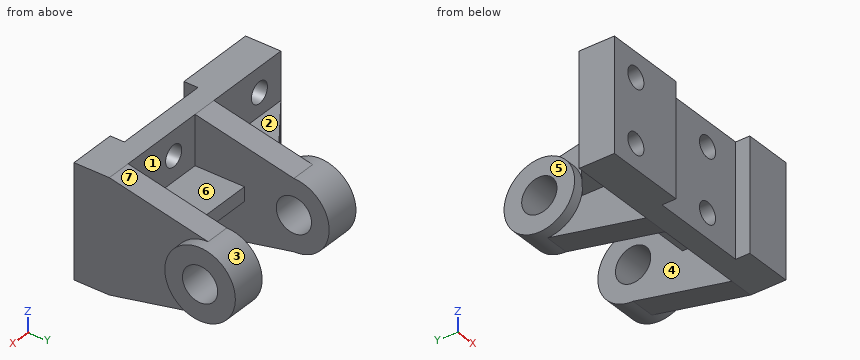
from build123d import *

# Parameters (mm, degrees)
SKETCH1_W           = 128
SKETCH1_H           = 64
BOSS_EXTRUDE1_DEPTH = 20
SKETCH2_W           = 55
SKETCH2_H           = 8
CUT_EXTRUDE1_DEPTH  = 93.69304181
SKETCH4_R           = 20
SKETCH4_R_2         = 10
BOSS_EXTRUDE3_DEPTH = 14
BOSS_EXTRUDE4_START = 6
SKETCH4_3_R         = 20
SKETCH4_3_R_2       = 10
BOSS_EXTRUDE4_DEPTH = 6
SKETCH18_W          = 50
SKETCH18_H          = 8
BOSS_EXTRUDE6_DEPTH = 28
RIB1_REACH          = 125.045
SKETCH19_WALL_W     = 309.701101848
SKETCH19_WALL_H     = 10
SKETCH20_R          = 6
CUT_EXTRUDE2_DEPTH  = 109.166538264
SKETCH21_R          = 6
CUT_EXTRUDE3_DEPTH  = 109.166538264
SKETCH22_R          = 6
CUT_EXTRUDE4_DEPTH  = 109.166538264


with BuildPart() as part:
    # Sketch1 → Boss-Extrude1 (new body)
    with BuildSketch(Plane(origin=(0, 0, 0), x_dir=(1, 0, 0), z_dir=(0, 1, 0))):
        Rectangle(SKETCH1_W, SKETCH1_H)
    extrude(amount=BOSS_EXTRUDE1_DEPTH)

    # Sketch2 → Cut-Extrude1 (cut, through all)
    with BuildSketch(Plane.XY.offset(32)):
        with Locations((9.5, 4)):
            Rectangle(SKETCH2_W, SKETCH2_H)
    extrude(amount=-CUT_EXTRUDE1_DEPTH, mode=Mode.SUBTRACT)

    # Sketch4 → Boss-Extrude3 (add)
    # profile 1 of 2: a face of its own
    with BuildSketch(Plane(origin=(64, 0, 0), x_dir=(0, 0, -1), z_dir=(1, 0, 0))):
        with BuildLine():
            ThreePointArc((20, 76), (0, 56), (-20, 76))
            Line((-20, 76), (-32, 20))
            Line((-32, 20), (32, 20))
            Line((32, 20), (20, 76))
        make_face()
    # profile 2 of 2: a face of its own
    with BuildSketch(Plane(origin=(64, 0, 0), x_dir=(0, 0, -1), z_dir=(1, 0, 0))):
        with Locations((0, 76)):
            Circle(SKETCH4_R)
        with Locations((0, 76)):
            Circle(SKETCH4_R_2, mode=Mode.SUBTRACT)
    boss_extrude3 = extrude(amount=-BOSS_EXTRUDE3_DEPTH)

    # Sketch4_3 → Boss-Extrude4 (add)
    with BuildSketch(Plane(origin=(64, 0, 0), x_dir=(0, 0, -1), z_dir=(1, 0, 0)).offset(BOSS_EXTRUDE4_START)):
        with Locations((0, 76)):
            Circle(SKETCH4_3_R)
        with Locations((0, 76)):
            Circle(SKETCH4_3_R_2, mode=Mode.SUBTRACT)
    boss_extrude4 = extrude(amount=-BOSS_EXTRUDE4_DEPTH)

    # Mirror2: Boss-Extrude3, Boss-Extrude4 across plane
    add(boss_extrude3.mirror(Plane.ZY.offset(-25)))
    add(boss_extrude4.mirror(Plane.ZY.offset(-25)))

    # Sketch18 → Boss-Extrude6 (add)
    with BuildSketch(Plane(origin=(0, 20, 0), x_dir=(1, 0, 0), z_dir=(0, 1, 0))):
        with Locations((25, 0)):
            Rectangle(SKETCH18_W, SKETCH18_H)
    extrude(amount=BOSS_EXTRUDE6_DEPTH)

    # Sketch19 wall → Rib1 (add, up to next)
    with BuildSketch(Plane(origin=(-39, 38, 0), x_dir=(0.811534341451, 0.584304725845, 0), z_dir=(-0.584304725845, 0.811534341451, 0)), mode=Mode.PRIVATE) as rib1_sk1:
        Rectangle(SKETCH19_WALL_W, SKETCH19_WALL_H)
    rib1_tool1 = extrude(rib1_sk1.sketch, amount=-RIB1_REACH, mode=Mode.PRIVATE) - part.part
    add(rib1_tool1.solids().sort_by_distance((-39, 38, 0))[0])

    # Sketch20 → Cut-Extrude2 (cut, through all)
    with BuildSketch(Plane(origin=(0, 20, 0), x_dir=(1, 0, 0), z_dir=(0, 1, 0))):
        with Locations(Location((16, -18, 0), (0, 0, 270))):
            Circle(SKETCH20_R)
    extrude(amount=-CUT_EXTRUDE2_DEPTH, mode=Mode.SUBTRACT)

    # Sketch21 → Cut-Extrude3 (cut, through all)
    with BuildSketch(Plane(origin=(0, 20, 0), x_dir=(1, 0, 0), z_dir=(0, 1, 0))):
        with Locations(Location((16, 18, 0), (0, 0, 270))):
            Circle(SKETCH21_R)
    extrude(amount=-CUT_EXTRUDE3_DEPTH, mode=Mode.SUBTRACT)

    # Sketch22 → Cut-Extrude4 (cut, through all)
    with BuildSketch(Plane(origin=(0, 20, 0), x_dir=(1, 0, 0), z_dir=(0, 1, 0))):
        with Locations(Location((-48, -18, 0), (0, 0, 270))):
            Circle(SKETCH22_R)
        with Locations(Location((-48, 18, 0), (0, 0, 270))):
            Circle(SKETCH22_R)
    extrude(amount=-CUT_EXTRUDE4_DEPTH, mode=Mode.SUBTRACT)


solid = part.part
For this review, take the finished solid that the model builds, in its own axes (mm). Face numbers are marked on the shaded views. A direction names the side the tool comes from. Round coordinates to 2 decimals unless told otherwise and drop trailing zeros. Order: outer loops, then holes, each group sorted by start corner. A loop starts at its lowest first (then second) coordinate and runs counter-clockwise, first axis right, second up. Notation, with made-up numbers: (-34, 83) -> (2, 83) arc R18 ccw to (2, 117) -> close; hole circle Ø7 at (-35, -20.75). An arc over 180 degrees is marked (long way). Write item = value, one per line. Start each with the question number.
1) Take a section at A-A on x = 16. State the section outline as (y, z) points.
2) Take a section at D-D on y = 69. State the section outline as (x, z) points (3 decimals).
3) Take a section at B-B on y = 17. State the section outline as (x, z) points.
4) Tool access review of the marked faces 1, 2, 3 and 4: name each direction out of +Z, -Z, +X, -X, +Y, -Y from which nothing blocks a thin tool from reaching the whole face with its end or side.
5) To check wall thickness, follow line 1 (X direction, y = 16.75, z = -18); line 2 (X direction, y = 45, z = -12.5); line 3 (X direction, y = 17, z = -4.5). State the ranges of each line that lie inside material, in increasing order. Write a range as from..to.
6) Take a section at C-C on z = 18. State the section outline as (x, y) points, plus the area to 3 significant figures.
7) Insertion check: pin 1 (11 mm diameter, centred on x = -35, y = 46, fed in from +Z); pin 2 (3 mm diameter, centred on x = -50.5, y = 29.5, fed in from -Z); pin 3 (1.5 mm diameter, centred on y = 45, z = -23.5, fed in from +X). Each pin has a flat end and moves straight along its axis. Give the tip position at first contact, or say it passes through.
8) The part is to be moulded in two halves that separate along X. For the marked faces 5, 6 and 7, say which applies: +X half, -X half, draft (parallel to the pull), parting line (faces both ways), or undercut.
Verdict:
q1.outline = (8, -32) -> (20, -32) -> (20, -24) -> (8, -24) -> close; (8, -12) -> (20, -12) -> (20, -4) -> (48, -4) -> (48, 4) -> (20, 4) -> (20, 12) -> (8, 12) -> close; (8, 24) -> (20, 24) -> (20, 32) -> (8, 32) -> close
q2.outline = (-20, -18.735) -> (-14, -18.735) -> (-14, -21.5) -> (0, -21.5) -> (0, -7.141) -> (-20, -7.141) -> close; (-20, 7.141) -> (0, 7.141) -> (0, 21.5) -> (-14, 21.5) -> (-14, 18.735) -> (-20, 18.735) -> close; (50, -21.5) -> (64, -21.5) -> (64, -18.735) -> (70, -18.735) -> (70, -7.141) -> (50, -7.141) -> close; (50, 7.141) -> (70, 7.141) -> (70, 18.735) -> (64, 18.735) -> (64, 21.5) -> (50, 21.5) -> close
q3.outline = (-64, -32) -> (64, -32) -> (64, 32) -> (-64, 32) -> close; hole circle Ø12 at (-48, -18); hole circle Ø12 at (-48, 18); hole circle Ø12 at (16, -18); hole circle Ø12 at (16, 18)
q4.face_1 = +Z, +Y
q4.face_2 = +Z, -X
q4.face_3 = +X
q4.face_4 = +Y
q5.line_1 = -64..-54, -42..10, 22..64
q5.line_2 = -14..0, 50..64
q5.line_3 = -64..64
q6.outline = (-64, 0) -> (-54, 0) -> (-54, 20) -> (-64, 20) -> close; (-42, 0) -> (-18, 0) -> (-18, 8) -> (10, 8) -> (10, 20) -> (0, 20) -> (0, 84.72) -> (-20, 84.72) -> (-20, 67.28) -> (-14, 67.28) -> (-14, 20) -> (-42, 20) -> close; (22, 8) -> (37, 8) -> (37, 0) -> (64, 0) -> (64, 67.28) -> (70, 67.28) -> (70, 84.72) -> (50, 84.72) -> (50, 20) -> (22, 20) -> close
q6.area = 3,760 mm2
q7.pin_1 = 5
q7.pin_2 = -5
q7.pin_3 = 64
q8.face_5 = -X half
q8.face_6 = undercut
q8.face_7 = draft
